from build123d import *

# Parameters (mm, degrees)
F1_FACE_R      = 7.5
F3_R           = 10
F6_D           = 6.5278
F6_CSINK_D     = 11
F6_CSINK_ANGLE = 82
F7_R           = 1


with BuildPart() as f1:
    # F0 (on Front) → F1 (revolve)
    with BuildSketch(Plane.XZ):
        Polygon((0, 5.5), (0, 0), (0, -5.5), (7.5, -5.5), (7.5, -2), (4, -2), (4, 0), (4, 2), (7.5, 2), (7.5, 5.5), align=None)
    revolve(axis=Axis((0, 0, 2.75), (0, 0, 1)))

    # F1_face (on face) → F4 section 0
    with BuildSketch(Plane(origin=(0, 0, -5.5), x_dir=(1, 0, 0), z_dir=(0, 0, -1))):
        Circle(F1_FACE_R)
    # F3 (on offset) → F4 section 1
    with BuildSketch(Plane(origin=(0, 0, -15.5), x_dir=(1, 0, 0), z_dir=(0, 0, -1))):
        Circle(F3_R)
    loft()

    # F6 (through all)
    with Locations(Plane.XY.offset(5.5)):
        with Locations((0, 0)):
            CounterSinkHole(F6_D / 2, F6_CSINK_D / 2, counter_sink_angle=F6_CSINK_ANGLE)

    # F7
    f7_edges = [f1.edges().sort_by_distance(p)[0] for p in [
        (-7.5, 0, 5.5),
    ]]
    fillet(f7_edges, radius=F7_R)


solid = f1.part
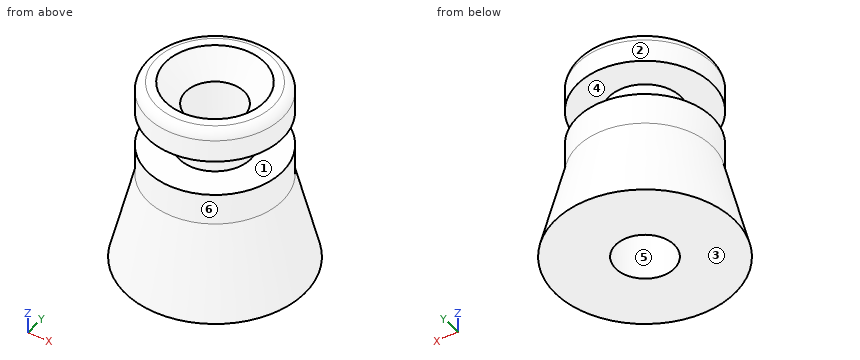
Verification items for the finished model (mm, model axes). Face numbers are marked on the shaded views. A direction names the side the tool comes from. Coordinates: 2 decimals unless noted, no trailing zeros. Order: outer loops, then holes, each group sorted by start corner. A loop starts at its lowest first (then second) coordinate and runs counter-clockwise, first axis right, second up. Notation, with made-up numbers: (-34, 19) -> (22, 19) arc R14 cw to (22, 40) -> close; hole circle Ø5 at (63, 59). An arc over 180 degrees is marked (long way). Put each result on its own line as item: value. Start each with the question number.
1. Cross-section at C-C, the plane z = 1.5. Record the boundary of the cut face in (x, y), then the cut area to 3 significant figures.
2. Go/stop test with flat-tipped pins: pin 1 Ø6 at (y, z) = (-4.5, -9.5) entering from +X; pin 2 Ø8 at (x, z) = (-7.5, -7.5) entering from +Y; pin 3 Ø4 at (x, z) = (7, -9) entering from +Y. Record where each tip stops, or that it passes through.
3. Cross-section at B-B, the plane z = -9.5. Record the boundary of the cut face in (x, y).
4. Access from +Z, -Z, +X, -X, +Y, -Y to the whole of each face (thin tool, end or side, straight path). Record for the marked faces 1, 2 and 3.
5. Cross-section at A-A, the plane x = 0. Record the boundary of the cut face in (y, z), then the cut area to 3 significant figures.
6. Material ranges on L1, parallel to Z at x = -5.75, y = -2.5; L2, parallel to Y at x = 0, z = -2.75; L3, parallel to X at y = 1, z = -8.5, recorded low to high. Write a range as [from, to].
7. Mould release check, pull along Y, two halves, no side actions. Record for the marked faces 4, 5 and 6: released by +Y, released by -Y, zero draft, split by the parting line, or undercut.
Computed:
1. outline: circle Ø8 at (0, 0); hole circle Ø6.53 at (0, 0)
1. area: 16.8 mm2
2. pin 1: x = 8.71
2. pin 2: y = 7.48
2. pin 3: y = 6.84
3. outline: circle Ø17 at (0, 0); hole circle Ø6.53 at (0, 0)
4. face 1: none
4. face 2: +Z
4. face 3: -Z, +X, -X, +Y, -Y
5. outline: (-10, -15.5) -> (-3.26, -15.5) -> (-3.26, 2.93) -> (-5.5, 5.5) -> (-6.5, 5.5) arc R1 ccw to (-7.5, 4.5) -> (-7.5, 2) -> (-4, 2) -> (-4, -2) -> (-7.5, -2) -> (-7.5, -5.5) -> close; (3.26, -15.5) -> (10, -15.5) -> (7.5, -5.5) -> (7.5, -2) -> (4, -2) -> (4, 2) -> (7.5, 2) -> (7.5, 4.5) arc R1 ccw to (6.5, 5.5) -> (5.5, 5.5) -> (3.26, 2.93) -> close
5. area: 169 mm2
6. L1: [-15.5, -2], [2, 5.5]
6. L2: [-7.5, -3.26], [3.26, 7.5]
6. L3: [-8.19, -3.11], [3.11, 8.19]
7. face 4: zero draft
7. face 5: undercut
7. face 6: split by the parting line
